Work out the finished part from the listing and answer in its coordinate system (mm). A direction names the side the tool comes from. Round coordinates to 2 decimals unless told otherwise and drop trailing zeros. Loops run counter-clockwise (first coordinate to the right, second up) from the corner with the lowest first, then second, coordinate; pieces in that order, holes last. Notation, with made-up numbers: (55.5, -25.5) -> (73.5, -25.5) arc R27 ccw to (73.5, -1.5) -> close; hole circle Ø11 at (-15, 8). An arc over 180 degrees is marked (long way). Use one line per item in the form item = value.
```python
from build123d import *

# Parameters (mm, degrees)
F0_W     = 25
F0_H     = 25
F1_DEPTH = 38
F2_W     = 20
F2_H     = 20
F3_DEPTH = 2
F5_DEPTH = 37


with BuildPart() as f1:
    # F0 (on Top) → F1 (new body)
    with BuildSketch(Plane.XY):
        with Locations((12.5, 12.5)):
            Rectangle(F0_W, F0_H)
    extrude(amount=F1_DEPTH)

    # F2 (on face) → F3 (join)
    with BuildSketch(Plane.XY.offset(38)):
        with Locations((12.5, 12.5)):
            Rectangle(F2_W, F2_H)
    extrude(amount=F3_DEPTH)

    # F4 (on face) → F5 (join)
    with BuildSketch(Plane.XY.offset(40)):
        with BuildLine():
            ThreePointArc((22.5, 2.7020410289), (25.4614813968, 7.2084973779), (26.5, 12.5))
            ThreePointArc((26.5, 12.5), (25.4614813968, 17.7915026221), (22.5, 22.2979589711))
            Line((22.5, 22.2979589711), (22.5, 2.7020410289))
        make_face()
        with BuildLine():
            Line((22.5, 2.7020410289), (22.5, 22.2979589711))
            ThreePointArc((22.5, 22.2979589711), (22.3994949366, 22.3994949366), (22.2979589711, 22.5))
            Line((22.2979589711, 22.5), (2.7020410289, 22.5))
            ThreePointArc((2.7020410289, 22.5), (2.6005050634, 22.3994949366), (2.5, 22.2979589711))
            Line((2.5, 22.2979589711), (2.5, 2.7020410289))
            ThreePointArc((2.5, 2.7020410289), (2.6005050634, 2.6005050634), (2.7020410289, 2.5))
            Line((2.7020410289, 2.5), (22.2979589711, 2.5))
            ThreePointArc((22.2979589711, 2.5), (22.3994949366, 2.6005050634), (22.5, 2.7020410289))
        make_face()
        with BuildLine():
            Line((2.7020410289, 22.5), (22.2979589711, 22.5))
            ThreePointArc((22.2979589711, 22.5), (12.5, 26.5), (2.7020410289, 22.5))
        make_face()
        with BuildLine():
            ThreePointArc((2.7020410289, 2.5), (12.5, -1.5), (22.2979589711, 2.5))
            Line((22.2979589711, 2.5), (2.7020410289, 2.5))
        make_face()
        with BuildLine():
            Line((2.5, 2.7020410289), (2.5, 22.2979589711))
            ThreePointArc((2.5, 22.2979589711), (-1.5, 12.5), (2.5, 2.7020410289))
        make_face()
    extrude(amount=F5_DEPTH)


solid = f1.part
```
(1) For a pull along Z with two mould halves and no side action, classify faces 5 (the flat face through (12, 24, 40)), 6 (the flat face through (12, 13, 77)), 7 (the flat face through (12, 25, 19)), 8 (the flat face through (22.5, 12, 39)) as +Z half, -Z half, draft (parallel to the pull), parting line (faces both ways), or undercut.
Completed:
face_5 = undercut
face_6 = +Z half
face_7 = draft
face_8 = undercut
(2) Find section C-C, the plane x = 18. Write down the section's boundary in (y, z).
Completed:
outline = (-0.37, 40) -> (2.5, 40) -> (2.5, 38) -> (0, 38) -> (0, 0) -> (25, 0) -> (25, 38) -> (22.5, 38) -> (22.5, 40) -> (25.37, 40) -> (25.37, 77) -> (-0.37, 77) -> close
(3) Find section A-A, the plane z = 52. Write down the section's boundary in (x, y), then the cut area to 3 significant figures.
Completed:
outline = circle Ø28 at (12.5, 12.5)
area = 616 mm2
(4) For faces 1 (the flat face through (12, 2.5, 39)), 2 (the flat face through (12, 22.5, 39)), 3 (the flat face through (23, 13, 38)), 4 (the flat face through (24, 13, 40)), determine the directions among +Z, -Z, +X, -X, +Y, -Y from which every point of the face is accessible in a straight line to the end or side of a thin tool.
Completed:
face_1 = +X, -X, -Y
face_2 = +X, -X, +Y
face_3 = none
face_4 = +X, +Y, -Y
(5) Find section B-B, the plane y = 4.5. Write down the section's boundary in (x, z).
Completed:
outline = (0, 0) -> (25, 0) -> (25, 38) -> (22.5, 38) -> (22.5, 40) -> (23.99, 40) -> (23.99, 77) -> (1.01, 77) -> (1.01, 40) -> (2.5, 40) -> (2.5, 38) -> (0, 38) -> close
(6) Find section D-D, the plane z = 5.5. Write down the section's boundary in (x, y).
Completed:
outline = (0, 0) -> (25, 0) -> (25, 25) -> (0, 25) -> close
(7) Consider L1, parallel to Z at x = 2.25, y = 18.25; L2, parallel to X at y = 11.25, z = 17.5. Determine where each line is inside the solid, lowest interval first.
Completed:
L1 = 0 to 38, 40 to 77
L2 = 0 to 25
(8) Given P1, Ø7.5, axis at y = 15, z = 15, coming from the -X side; P2, Ø4, axis at x = 8.5, z = 16, coming from the -Y side; P3, Ø0.6, axis at y = 16.5, z = 39.5, coming from the -X side, each flat-ended and moving along its own axis, determine where each tip first touches the part or whether it passes through.
Completed:
P1 = 0
P2 = 0
P3 = 2.5
